Geometry: final body of the model. Coordinates: model frame, mm. Give positions to 0.01 mm unless a question says otherwise; leave off trailing zeros. Write each loop counter-clockwise with the first axis right and the second up, starting at its lowest first coordinate (ties: lowest second). Pieces come first, ordered by that corner, then holes. Notation, with made-up numbers: (-15, 80) -> (41, 80) arc R24 ccw to (41, 94) -> close; hole circle Ø7 at (-38.5, -16.5). An arc over 180 degrees is marked (long way). Answer as a JSON object with one key per item and string values. Group by question number.
(1) Section query A-A on y = 35. Output: boundary loops of the cut face in (x, z).
(2) Contact query for a flat-ended pin moving along its axis: pin 1 Ø1.8 at (x, y) = (0, -35) entering from +Z. Output: stop coordinate, or through.
(3) Section query C-C on z = 1.55. Output: boundary loops of the cut face in (x, y), plus the area to 3 significant figures.
(4) Draft query along X for faces 1 (the face through (-0.325, 33.536, 2.535)), 2 (the face through (-3.43, 39.4, 2.54)), 3 (the face through (0, -40, 2)). Return one class per face: +X half, -X half, draft (parallel to the pull), parting line (faces both ways), or undercut.
(5) Section query B-B on x = 0. Output: boundary loops of the cut face in (y, z).
(6) Material intervals for probe 1 along Y at (x, z) = (0, 2.25); probe 2 along Y at (x, z) = (2.5, 0.35); probe 3 along Y at (x, z) = (3.5, 0.9), sorted ascending.
from build123d import *

# Parameters (mm, degrees)
SKETCH_1_W          = 8
SKETCH_1_H          = 80
EXTRUDE_1_DEPTH     = 5
SKETCH_2_R          = 1.5
CUT_EXTRUDE_1_DEPTH = 41.509258201
FILLET_1_R          = 2


with BuildPart() as part:
    # 草图1 → 凸台-拉伸1 (new body)
    with BuildSketch(Plane.XY):
        Rectangle(SKETCH_1_W, SKETCH_1_H)
    extrude(amount=EXTRUDE_1_DEPTH)

    # 草图2 → 切除-拉伸1 (cut, through all)
    with BuildSketch(Plane.XY.offset(5)):
        with Locations((0, 35)):
            Circle(SKETCH_2_R)
        with Locations((0, -35)):
            Circle(SKETCH_2_R)
    extrude(amount=-CUT_EXTRUDE_1_DEPTH, mode=Mode.SUBTRACT)

    # 圆角1
    fillet_1_edges = [part.edges().sort_by_distance(p)[0] for p in [
        (-4, 40, 2.5),
        (4, 40, 2.5),
        (4, -40, 2.5),
        (-4, -40, 2.5),
    ]]
    fillet(fillet_1_edges, radius=FILLET_1_R)


solid = part.part
Answer list:
{
 "1": {"outline": "(-4, 0) -> (-1.5, 0) -> (-1.5, 5) -> (-4, 5) -> close; (1.5, 0) -> (4, 0) -> (4, 5) -> (1.5, 5) -> close"},
 "2": {"pin 1": "through"},
 "3": {"outline": "(-4, -38) arc R2 ccw to (-2, -40) -> (2, -40) arc R2 ccw to (4, -38) -> (4, 38) arc R2 ccw to (2, 40) -> (-2, 40) arc R2 ccw to (-4, 38) -> close; hole circle Ø3 at (0, -35); hole circle Ø3 at (0, 35)", "area": "622 mm2"},
 "4": {"face 1": "undercut", "face 2": "-X half", "face 3": "draft"},
 "5": {"outline": "(-40, 0) -> (-36.5, 0) -> (-36.5, 5) -> (-40, 5) -> close; (-33.5, 0) -> (33.5, 0) -> (33.5, 5) -> (-33.5, 5) -> close; (36.5, 0) -> (40, 0) -> (40, 5) -> (36.5, 5) -> close"},
 "6": {"probe 1": "-40 to -36.5, -33.5 to 33.5, 36.5 to 40", "probe 2": "-39.94 to 39.94", "probe 3": "-39.32 to 39.32"}
}
